```python
from build123d import *

# Parameters (mm, degrees)
CUT_EXTRUDE1_REACH             = 33.75
SKETCH2_W                      = 19.05
SKETCH2_H                      = 64.439050054
CUT_EXTRUDE1_DIRECTION_2_DEPTH = 32.7500001
SKETCH3_W                      = 12
SKETCH3_H                      = 21
CUT_EXTRUDE2_DEPTH             = 8
SKETCH4_R                      = 4
CUT_EXTRUDE3_DEPTH             = 6.9700001
SKETCH7_W                      = 19.05
SKETCH7_H                      = 5
CUT_EXTRUDE4_DEPTH             = 5


with BuildPart() as part:
    # Sketch1 → Revolve1 (revolve)
    with BuildSketch(Plane.XY):
        with BuildLine():
            Line((-9.525, 0), (-9.525, -17.78))
            Line((-9.525, -17.78), (9.525, -17.78))
            Line((9.525, -17.78), (9.525, 0))
            add(Edge.make_bspline(
                [(9.525, 0), (9.525, 13.97), (0, 13.97), (-9.525, 13.97), (-9.525, 0)],
                knots=[1.570796327, 1.570796327, 1.570796327, 3.141592654, 3.141592654, 4.71238898, 4.71238898, 4.71238898], degree=2, weights=[1, 0.707106781, 1, 0.707106781, 1]))
        make_face()
    revolve(axis=Axis((-20.584458519, -17.78, 0), (1, 0, 0)))

    # Sketch2 → Cut-Extrude1 (cut, up to next)
    with BuildSketch(Plane.XY, mode=Mode.PRIVATE) as cut_extrude1_sk1:
        with Locations((0, -32.219525027)):
            Rectangle(SKETCH2_W, SKETCH2_H)
    cut_extrude1_tool1 = extrude(cut_extrude1_sk1.sketch, amount=-CUT_EXTRUDE1_REACH, mode=Mode.PRIVATE) & part.part
    add(cut_extrude1_tool1.solids().sort_by_distance((0, -32.219525, 0))[0], mode=Mode.SUBTRACT)

    # Sketch2 → Cut-Extrude1 direction 2 (cut)
    with BuildSketch(Plane.XY):
        with Locations((0, -32.219525027)):
            Rectangle(SKETCH2_W, SKETCH2_H)
    extrude(amount=CUT_EXTRUDE1_DIRECTION_2_DEPTH, mode=Mode.SUBTRACT)

    # Sketch3 → Cut-Extrude2 (cut)
    with BuildSketch(Plane.XZ):
        Rectangle(SKETCH3_W, SKETCH3_H)
    extrude(amount=-CUT_EXTRUDE2_DEPTH, mode=Mode.SUBTRACT)

    # Sketch4 → Cut-Extrude3 (cut, through all)
    with BuildSketch(Plane.XZ.offset(-8)):
        with Locations((0, 4.5)):
            Circle(SKETCH4_R)
    extrude(amount=-CUT_EXTRUDE3_DEPTH, mode=Mode.SUBTRACT)

    # Sketch5 → Cut-Revolve1 (revolve, cut)
    with BuildSketch(Plane(origin=(0, 0, 0), x_dir=(0, 0, -1), z_dir=(1, 0, 0))):
        Polygon((-16.05, 13.97), (-16.05, 2.032), (-17.145, 2.032), (-17.145, 0), (-19.05, 0), (-19.05, 13.97), align=None)
    cut_revolve1 = revolve(axis=Axis((0, 0, 19.05), (0, -1, 0)), mode=Mode.SUBTRACT)

    # Mirror1: Cut-Revolve1 across plane
    add(cut_revolve1.mirror(Plane.XY), mode=Mode.SUBTRACT)

    # Sketch6 → Cut-Revolve2 (revolve, cut)
    with BuildSketch(Plane(origin=(0, 0, 0), x_dir=(0, 0, -1), z_dir=(1, 0, 0))):
        Polygon((3, 13.97), (3, 9.524), (4.095, 9.524), (4.095, 0), (6, 0), (6, 13.97), align=None)
    revolve(axis=Axis((0, 0, -6), (0, -1, 0)), mode=Mode.SUBTRACT)

    # Sketch7 → Cut-Extrude4 (cut)
    with BuildSketch(Plane.XZ):
        with Locations((0, -13)):
            Rectangle(SKETCH7_W, SKETCH7_H)
    extrude(amount=-CUT_EXTRUDE4_DEPTH, mode=Mode.SUBTRACT)


solid = part.part
```
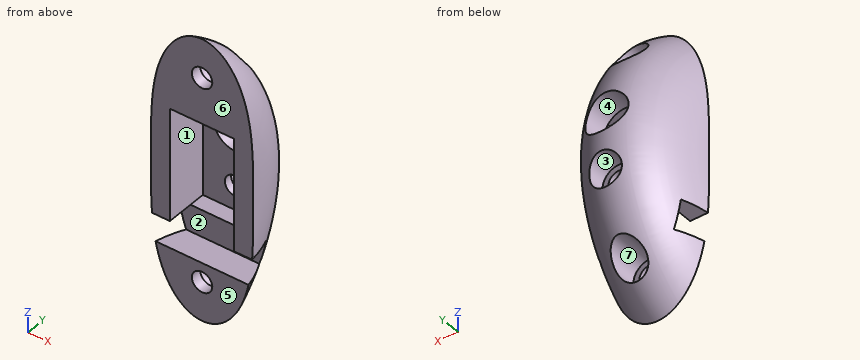
Check sheet for the modelled part. Datum: model origin and axes. Units: mm. Face numbers are marked on the shaded views. A direction names the side the tool comes from. Round coordinates to 2 decimals unless told otherwise and drop trailing zeros. Write item = value, one per line. Start each with the question number.
1) Gauge pin test, flat ends, axial feed: pin 1 Ø1.8 at (x, z) = (0, -19.5) entering from +Y; pin 2 Ø10 at (x, z) = (-1.5, 14) entering from -Y; pin 3 Ø3.5 at (x, y) = (-7.5, 3.5) entering from -Z; pin 4 Ø6.5 at (x, z) = (-0.5, -4.5) entering from +Y. Record the tip position at first contact, or that the pin passes through.
2) Release check for a two-part mould opening along Z. For the marked faces 6 and 7 record: released by +Z, released by -Z, zero draft, split by the parting line, or undercut.
3) Sectioned sample at A-A, the plane y = 4. State how many separate pieces and enclosed holes the cut face has, plus the area to 3 significant figures.
4) Set-up check for the marked faces 1, 2, 3, 4 and 5: record each of +Z, -Z, +X, -X, +Y, -Y from which the full face is reachable in a straight line by a thin tool's end or side.
5) Thickness scan on probe 1 along Z at (x, y) = (2.5, 10.25); probe 2 along X at (y, z) = (12.35, -6); probe 3 along Z at (x, y) = (0, 2.5). Record the ranges inside material, lowest first.
Results are:
q1.pin_1 = through
q1.pin_2 = 0
q1.pin_3 = -20.11
q1.pin_4 = 13.94
q2.face_6 = zero draft
q2.face_7 = undercut
q3.separate_pieces = 2
q3.enclosed_holes = 2
q3.area = 304 mm^2
q4.face_1 = -Y
q4.face_2 = +X, -X, -Y
q4.face_3 = +Y
q4.face_4 = +Y, -Y
q4.face_5 = +Z, -Z, +X, -X, -Y
q5.probe_1 = -13.84 to -7.66, -4.34 to 1.38, 7.62 to 13.84
q5.probe_2 = -3.59 to -3, 3 to 3.59
q5.probe_3 = -24.43 to -22.05, -16.05 to -15.5, 10.5 to 16.05, 22.05 to 24.43
